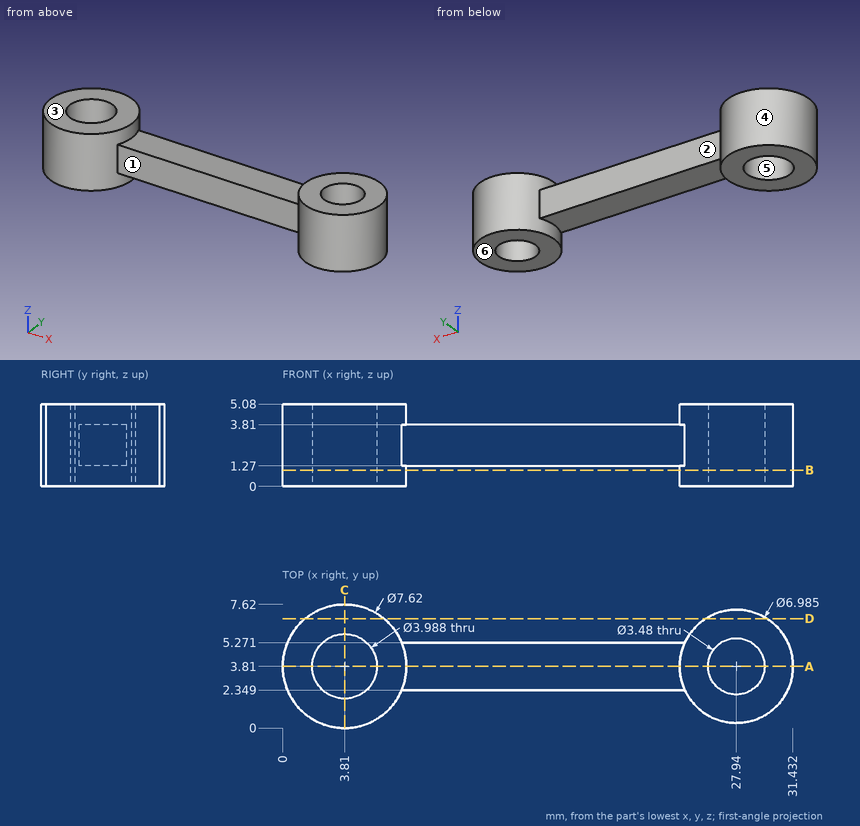
Design review of the part shown in the three views and the two pictorial views. Dimensions are in mm from the part's minimum x, y and z. A direction names the side the tool comes from. Round coordinates to 2 decimals unless told otherwise and drop trailing zeros. Order: outer loops, then holes, each group sorted by start corner. A loop starts at its lowest first (then second) coordinate and runs counter-clockwise, first axis right, second up. Notation, with made-up numbers: (20.25, 56.25) - (67.25, 56.25) arc R20 ccw to (67.25, 93.25) - close; hole circle Ø1 at (-33.75, -35.5). An arc over 180 degrees is marked (long way). One line per question, with ' | ' between items.
Item 1: Take a section at B-B, the plane z = 1. Write out the cut boundary in (x, y) (1 decimal).
Checks:
outline: circle Ø7.6 at (3.8, 3.8); circle Ø7 at (27.9, 3.8); hole circle Ø4 at (3.8, 3.8); hole circle Ø3.5 at (27.9, 3.8)
Item 2: Take a section at D-D, the plane y = 6.75. Write out the cut boundary in (x, z) (1 decimal).
Checks:
outline: (1.4, 0) - (6.2, 0) - (6.2, 5.1) - (1.4, 5.1) - close; (26.1, 0) - (29.8, 0) - (29.8, 5.1) - (26.1, 5.1) - close
Item 3: Machinability: for the marked faces 1, 2 and 3, which of the approach directions +Z, -Z, +X, -X, +Y, -Y give a long, thin tool a straight path to every point of the face, cutting with its end or side? Answer none if there is none.
Checks:
face 1: +Z, -Z, -Y | face 2: +Z, -Z, +Y | face 3: +Z, +X, -X, +Y, -Y
Item 4: Take a section at A-A, the plane y = 3.81. Write out the cut boundary in (x, z).
Checks:
outline: (0, 0) - (1.82, 0) - (1.82, 5.08) - (0, 5.08) - close; (5.8, 0) - (7.62, 0) - (7.62, 1.27) - (24.45, 1.27) - (24.45, 0) - (26.2, 0) - (26.2, 5.08) - (24.45, 5.08) - (24.45, 3.81) - (7.62, 3.81) - (7.62, 5.08) - (5.8, 5.08) - close; (29.68, 0) - (31.43, 0) - (31.43, 5.08) - (29.68, 5.08) - close
Item 5: Wall thickness on line 1 (X direction, y = 3.81, z = 1.1); line 2 (Y direction, x = 3.81, z = 1.9); line 3 (Y direction, x = 27.94, z = 1.3): over which ranges is each line inside the solid? List them lowest first. Write a range as [from, to].
Checks:
line 1: [0, 1.82], [5.8, 7.62], [24.45, 26.2], [29.68, 31.43] | line 2: [0, 1.82], [5.8, 7.62] | line 3: [0.32, 2.07], [5.55, 7.3]
Item 6: Draft analysis for pull direction X (two halves, no side actions). For the marked faces 4, 5 and 6, state which applies: +X half, -X half, draft (parallel to the pull), parting line (faces both ways), or undercut.
Checks:
face 4: undercut | face 5: undercut | face 6: draft
Item 7: For P1, Ø0.8, axis at x = 18, z = 2, coming from the +Y side; P2, Ø3, axis at x = 27.94, y = 3.81, coming from the +Z side; P3, Ø1.5, axis at y = 6, z = 4.5, coming from the +X side; P4, Ø0.9, axis at x = 19, y = 3.5, coming from the -Z side, all flat-tipped, find the tip position at first contact; note any pin that passes through.
Checks:
P1: y = 5.27 | P2: through | P3: x = 31.12 | P4: z = 1.27
Item 8: Take a section at C-C, the plane x = 3.81. Write out the cut boundary in (y, z).
Checks:
outline: (0, 0) - (1.82, 0) - (1.82, 5.08) - (0, 5.08) - close; (5.8, 0) - (7.62, 0) - (7.62, 5.08) - (5.8, 5.08) - close
